Read the model definition and answer for the solid it produces. Units are mm, in the model's axes. Coordinates: 2 decimals unless noted, no trailing zeros. Write each loop counter-clockwise with the first axis right and the second up, starting at its lowest first coordinate (ties: lowest second). Pieces come first, ordered by that corner, then holes.
Item 1: Section C-C (x = 26) is taken. Give the vertices of the cut face in (y, z), then the cut area to 3 significant figures.
Item 2: Section A-A (z = 67.5) is taken. Give the vertices of the cut face in (x, y), then the cut area to 3 significant figures.
Item 3: Straight lines are drawn through the part: probe 1 along X at (y, z) = (46.5, 56); probe 2 along Z at (x, y) = (49.5, 45.5); probe 3 along Z at (x, y) = (20, 45). For each, find the intervals that lie inside material, in ascending order.
Item 4: Section B-B (y = 44) is taken. Give the vertices of the cut face in (x, z), then the cut area to 3 significant figures.
Item 5: Each of these flat-tipped pins is pushed along its axis until it touches: P1, Ø7, axis at x = 69.41, y = 22.94, coming from the +Z side; P2, Ø5, axis at y = 39, z = 68.5, coming from the -X side; P3, Ø11, axis at y = 21, z = -2.5, coming from the -X side; P4, Ø9.5, axis at x = 8.86, y = 12.9, coming from the -Z side. Where does it stop, or does it pass through?
from build123d import *

# Parameters (mm, degrees)
ESQUISSE1_R             = 3
BOSS_EXTRU_1_DEPTH      = 200
ESQUISSE4_W             = 5
ESQUISSE4_H             = 50
BOSS_EXTRU_4_DEPTH      = 180
BOSS_EXTRU_7_DEPTH      = 50
ESQUISSE6_W             = 20
ESQUISSE6_H             = 10.719834163
ENL_V_MAT_EXTRU_2_DEPTH = 10
ESQUISSE5_W             = 10
ESQUISSE5_H             = 10
ENL_V_MAT_EXTRU_1_DEPTH = 10
ESQUISSE14_R            = 5
ENL_V_MAT_EXTRU_4_DEPTH = 15
BOSS_EXTRU_8_REACH      = 242.401
ESQUISSE16_W            = 219.108996988
ESQUISSE16_H            = 68.482817494
ENL_V_MAT_EXTRU_5_DEPTH = 105


with BuildPart() as part:
    # Esquisse1 → Boss.-Extru.1 (new body)
    with BuildSketch(Plane.XY):
        Polygon((-105.796013405, 0), (84.203986595, 0), (84.203986595, 33.502126335), (-105.796013405, 2), align=None)
        with Locations((69.406004871, 22.939397164)):
            Circle(ESQUISSE1_R, mode=Mode.SUBTRACT)
        with Locations((40.981469067, 6.77616521)):
            Circle(ESQUISSE1_R, mode=Mode.SUBTRACT)
        with Locations((-40.796013405, 6)):
            Circle(ESQUISSE1_R, mode=Mode.SUBTRACT)
        with Locations((8.861542866, 12.901085106)):
            Circle(ESQUISSE1_R, mode=Mode.SUBTRACT)
    extrude(amount=BOSS_EXTRU_1_DEPTH)

    # Esquisse4 → Boss.-Extru.4 (add)
    with BuildSketch(Plane(origin=(84.203986595, 0, 0), x_dir=(0, 0, -1), z_dir=(1, 0, 0))):
        with Locations((-202.5, 25)):
            Rectangle(ESQUISSE4_W, ESQUISSE4_H)
        with Locations((2.5, 25)):
            Rectangle(ESQUISSE4_W, ESQUISSE4_H)
    extrude(amount=-BOSS_EXTRU_4_DEPTH)

    # Esquisse8 → Boss.-Extru.7 (add)
    with BuildSketch(Plane(origin=(0, 50, 0), x_dir=(1, 0, 0), z_dir=(0, 1, 0))):
        Polygon((84.203986595, 0), (-95.796013405, 0), (-95.796013405, -5), align=None)
    boss_extru_7 = extrude(amount=-BOSS_EXTRU_7_DEPTH)

    # Esquisse6 → Enlèv. mat.-Extru.2 (cut)
    with BuildSketch(Plane(origin=(0, 0, -5), x_dir=(-1, 0, 0), z_dir=(0, 0, -1))):
        with Locations((95.796013405, 5.359917081)):
            Rectangle(ESQUISSE6_W, ESQUISSE6_H)
    enl_v_mat_extru_2 = extrude(amount=-ENL_V_MAT_EXTRU_2_DEPTH, mode=Mode.SUBTRACT)

    # Esquisse5 → Enlèv. mat.-Extru.1 (cut)
    with BuildSketch(Plane(origin=(84.203986595, 0, 0), x_dir=(0, 0, -1), z_dir=(1, 0, 0))):
        with Locations((-200, 5)):
            Rectangle(ESQUISSE5_W, ESQUISSE5_H)
        with Locations((0, 5)):
            Rectangle(ESQUISSE5_W, ESQUISSE5_H)
    extrude(amount=-ENL_V_MAT_EXTRU_1_DEPTH, mode=Mode.SUBTRACT)

    # Esquisse14 → Enlèv. mat.-Extru.4 (cut)
    with BuildSketch(Plane(origin=(0, 0, -5), x_dir=(-1, 0, 0), z_dir=(0, 0, -1))):
        with Locations((-69.406004871, 22.939397164)):
            Circle(ESQUISSE14_R)
        with Locations((-40.981469067, 6.77616521)):
            Circle(ESQUISSE14_R)
        with Locations((-8.861542866, 12.901085106)):
            Circle(ESQUISSE14_R)
        with Locations((40.796013405, 6)):
            Circle(ESQUISSE14_R)
    enl_v_mat_extru_4 = extrude(amount=-ENL_V_MAT_EXTRU_4_DEPTH, mode=Mode.SUBTRACT)

    # Symétrie3: Boss.-Extru.7, Enlèv. mat.-Extru.2, Enlèv. mat.-Extru.4 across plane
    add(boss_extru_7.mirror(Plane(origin=(0, 0, 100), x_dir=(1, 0, 0), z_dir=(0, 0, -1))))
    add(enl_v_mat_extru_2.mirror(Plane(origin=(0, 0, 100), x_dir=(1, 0, 0), z_dir=(0, 0, -1))), mode=Mode.SUBTRACT)
    add(enl_v_mat_extru_4.mirror(Plane(origin=(0, 0, 100), x_dir=(1, 0, 0), z_dir=(0, 0, -1))), mode=Mode.SUBTRACT)

    # Boss.-Extru.8: up to this plane
    boss_extru_8_end = Plane(origin=(-95.796013405, -180.069431054, 195), z_dir=(-0.0277670672403533, 0, 0.9996144206527183))
    # Esquisse15 → Boss.-Extru.8 (add, up to the surface)
    with BuildSketch(Plane(origin=(0, 0, -5), x_dir=(-1, 0, 0), z_dir=(0, 0, -1)), mode=Mode.PRIVATE) as boss_extru_8_sk1:
        Polygon((-84.203986595, 33.502126335), (-79.203986595, 32.67312301), (-79.203986595, 50), (-84.203986595, 50), align=None)
    boss_extru_8_tool1 = split(extrude(boss_extru_8_sk1.sketch, amount=-BOSS_EXTRU_8_REACH, mode=Mode.PRIVATE), bisect_by=boss_extru_8_end, keep=Keep.BOTH, mode=Mode.PRIVATE)
    add(boss_extru_8_tool1.solids().sort_by_distance((81.683563, 41.542119, -5))[0])

    # Esquisse16 → Enlèv. mat.-Extru.5 (cut)
    with BuildSketch(Plane(origin=(0, 0, 100), x_dir=(-1, 0, 0), z_dir=(0, 0, -1))):
        with Locations((5.796013405, 28.916172848)):
            Rectangle(ESQUISSE16_W, ESQUISSE16_H)
    extrude(amount=-ENL_V_MAT_EXTRU_5_DEPTH, mode=Mode.SUBTRACT)


solid = part.part
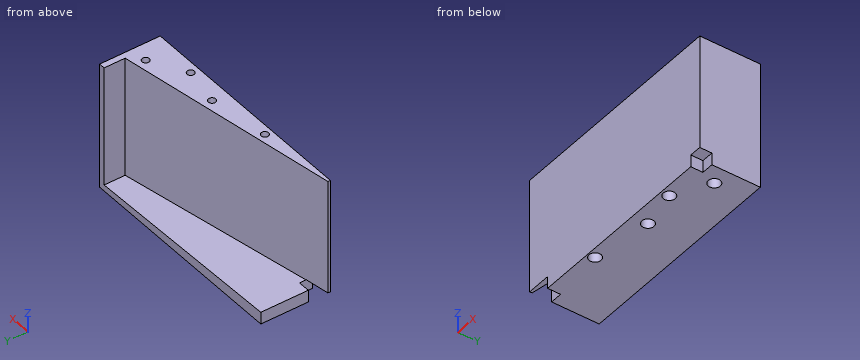
Established:
1. outline: (0, -5) - (50, -5) - (50, 1.62) - (23.85, 1.62) - (23.85, 100) - (0, 100) - close
1. area: 2,680 mm2
2. outline: (-105.8, 0) - (84.2, 0) - (84.2, 50) - (79.2, 50) - (79.2, 32.67) - (-105.8, 2) - close; hole circle Ø6 at (-40.8, 6); hole circle Ø6 at (8.86, 12.9); hole circle Ø6 at (40.98, 6.78); hole circle Ø6 at (69.41, 22.94)
2. area: 3,340 mm2
3. probe 1: x = 79.2 to 84.2
3. probe 2: z = -5 to 0.96
3. probe 3: z = -5 to 1.78
4. outline: (-95.8, -5) - (84.2, -5) - (84.2, 100) - (79.2, 100) - (79.2, 0.14) - (-95.8, 5) - close
4. area: 1,850 mm2
5. P1: stops at z = 100
5. P2: stops at x = 79.2
5. P3: stops at x = -95.8
5. P4: stops at z = 10
